Geometry: final body of the model. Coordinates: model frame, mm. Face numbers are marked on the shaded views. A direction names the side the tool comes from. Give positions to 0.01 mm unless a question says otherwise; leave off trailing zeros. Loops run counter-clockwise (first coordinate to the right, second up) from the corner with the lowest first, then second, coordinate; pieces in that order, holes last.
1. Section B-B, the plane z = 24. Output: boundary loops of the cut face in (x, y).
2. Draft query along X for the marked faces 4, 5 and 6. Return one class per face: +X half, -X half, draft (parallel to the pull), parting line (faces both ways), or undercut.
3. Section A-A, the plane y = -21. Output: boundary loops of the cut face in (x, z), then the cut area to 3 significant figures.
4. First-contact query: P1, Ø1.2, axis at x = 42.5, y = -35.5, coming from the -Z side; P2, Ø3.5, axis at x = 35, z = 34, coming from the -Y side; P3, Ø1.5, axis at x = -19.5, z = 66.5, coming from the +Y side. Flat tips, straight axial feed; report the tip coordinate or a pass-through.
5. Access query for the marked faces 1, 2 and 3. Directions: +Z, -Z, +X, -X, +Y, -Y. A direction counts if a zero-diameter tool reaches every point of the face in a straight line with its end or side. Return the directions, or none.
6. Material intervals for line 1 along Z through (x, y) = (43, -44); line 2 along Z through (x, y) = (7, -14.75); line 3 along Z through (x, y) = (40, -1.75), sorted ascending.
7. Section C-C, the plane x = -22. Output: boundary loops of the cut face in (y, z), then the cut area to 3 significant figures.
8. Section D-D, the plane z = 55. Output: boundary loops of the cut face in (x, y).
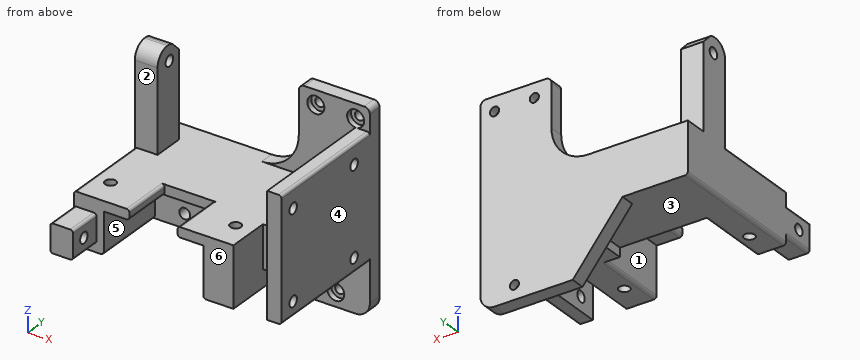
from build123d import *

# Parameters (mm, degrees)
PAD_DEPTH            = 70
SKETCH001_W          = 11.887794
SKETCH001_H          = 46.78
POCKET_DEPTH         = 70.001
POCKET001_DEPTH      = 30
SKETCH003_R          = 1.9
POCKET002_DEPTH      = 40.001
SKETCH004_W          = 17
SKETCH004_H          = 23.314381
POCKET003_DEPTH      = 40.001
SKETCH005_W          = 35
SKETCH005_H          = 57.974789
POCKET004_DEPTH      = 26
SKETCH006_W          = 45.255611
SKETCH006_H          = 30.428207
POCKET005_DEPTH      = 28
POCKET005_DEPTH_BACK = -100
SKETCH007_W          = 26.242121
SKETCH007_H          = 29.741062
POCKET006_DEPTH      = 45
SKETCH008_W          = 15.625622
SKETCH008_H          = 14.392597
SKETCH008_W_2        = 24.610352
SKETCH008_H_2        = 31.67345
POCKET007_DEPTH      = 45
SKETCH009_R          = 1.9
POCKET008_DEPTH      = 13
SKETCH010_R          = 1.6
POCKET009_DEPTH      = 5
SKETCH014_W          = 10
SKETCH014_H          = 15
PAD001_DEPTH         = 23
SKETCH015_W          = 11
SKETCH015_H          = 38.184422
SKETCH015_W_2        = 19.881198
SKETCH015_H_2        = 10
PAD002_DEPTH         = 8
SKETCH013_R          = 1.9
POCKET010_DEPTH      = 17
SKETCH011_R          = 1.9
POCKET011_DEPTH      = 15
PAD003_DEPTH         = 5
SKETCH017_R          = 3
POCKET012_DEPTH      = 2
CHAMFER_SIZE         = 4
FILLET_R             = 5
FILLET001_R          = 1
FILLET002_R          = 1
FILLET003_R          = 1
FILLET004_R          = 1
FILLET005_R          = 5
FILLET006_R          = 1
FILLET007_R          = 2
FILLET008_R          = 1
FILLET009_R          = 13
FILLET010_R          = 1
FILLET011_R          = 3


with BuildPart() as part:
    # Sketch → Pad (new body)
    with BuildSketch(Plane.XY):
        Polygon((0, 0), (45, 0), (45, -50), (-28, -50), (-28, 0), align=None)
    extrude(amount=PAD_DEPTH)

    # Sketch001 (on Face7 of Pad) → Pocket (cut, through all)
    with BuildSketch(Plane.XY.offset(70)):
        with Locations((34.056103, -28.39)):
            Rectangle(SKETCH001_W, SKETCH001_H)
    extrude(amount=-POCKET_DEPTH, mode=Mode.SUBTRACT)

    # Sketch002 (on Face5 of Pocket) → Pocket001 (cut)
    with BuildSketch(Plane.XY.offset(70)):
        Polygon((30, -5), (30, -65.096024), (-40.783405, -65.096024), (-40.783405, 12.994774), (20, 12.994774), (20, -5), align=None)
    extrude(amount=-POCKET001_DEPTH, mode=Mode.SUBTRACT)

    # Sketch003 (on Face6 of Pocket001) → Pocket002 (cut, through all)
    with BuildSketch(Plane.XY.offset(40)):
        with Locations((-22, -40)):
            Circle(SKETCH003_R)
        with Locations((22, -40)):
            Circle(SKETCH003_R)
    extrude(amount=-POCKET002_DEPTH, mode=Mode.SUBTRACT)

    # Sketch004 (on Face6 of Pocket002) → Pocket003 (cut, through all)
    with BuildSketch(Plane.XY.offset(40)):
        with Locations((0, -43.65719)):
            Rectangle(SKETCH004_W, SKETCH004_H)
    extrude(amount=-POCKET003_DEPTH, mode=Mode.SUBTRACT)

    # Sketch005 (on Face13 of Pocket003) → Pocket004 (cut)
    with BuildSketch(Plane.XZ.offset(50)):
        with Locations((0, 7.512606)):
            Rectangle(SKETCH005_W, SKETCH005_H)
    extrude(amount=-POCKET004_DEPTH, mode=Mode.SUBTRACT)

    # Sketch006 (on Face11 of Pocket004) → Pocket005 (cut, two sides)
    with BuildSketch(Plane.XZ.offset(24)) as pocket005_sk:
        with Locations((-10.127806, 6.785896)):
            Rectangle(SKETCH006_W, SKETCH006_H)
    extrude(amount=-POCKET005_DEPTH, mode=Mode.SUBTRACT)
    extrude(pocket005_sk.sketch, amount=-POCKET005_DEPTH_BACK, mode=Mode.SUBTRACT)

    # Sketch007 (on Face12 of Pocket005) → Pocket006 (cut)
    with BuildSketch(Plane.XZ.offset(50)):
        with Locations((20.733142, 3.968048)):
            Rectangle(SKETCH007_W, SKETCH007_H)
    extrude(amount=-POCKET006_DEPTH, mode=Mode.SUBTRACT)

    # Sketch008 (on Face14 of Pocket006) → Pocket007 (cut)
    with BuildSketch(Plane.XZ.offset(50)):
        with Locations((42.909006, 69.196298)):
            Rectangle(SKETCH008_W, SKETCH008_H)
        with Locations((46.359665, 3.163275)):
            Rectangle(SKETCH008_W_2, SKETCH008_H_2)
    extrude(amount=-POCKET007_DEPTH, mode=Mode.SUBTRACT)

    # Sketch009 (on Face3 of Pocket007) → Pocket008 (cut)
    with BuildSketch(Plane.YZ.offset(45)):
        with Locations((-44, 55)):
            Circle(SKETCH009_R)
        with Locations((-13, 24)):
            Circle(SKETCH009_R)
        with Locations((-13, 55)):
            Circle(SKETCH009_R)
        with Locations((-44, 24)):
            Circle(SKETCH009_R)
    extrude(amount=-POCKET008_DEPTH, mode=Mode.SUBTRACT)

    # Sketch010 (on Face1 of Pocket008) → Pocket009 (cut)
    with BuildSketch(Plane(origin=(0, 0, 0), x_dir=(-1, 0, 0), z_dir=(0, 1, 0))):
        with Locations((-33, 5)):
            Circle(SKETCH010_R)
        with Locations((-40, 65)):
            Circle(SKETCH010_R)
        with Locations((-26, 65)):
            Circle(SKETCH010_R)
    extrude(amount=-POCKET009_DEPTH, mode=Mode.SUBTRACT)

    # Sketch014 (on Face4 of Pocket009) → Pad001 (join)
    with BuildSketch(Plane.YZ.offset(45)):
        with Locations((-30, 32.5)):
            Rectangle(SKETCH014_W, SKETCH014_H)
    extrude(amount=-PAD001_DEPTH)

    # Sketch015 (on Face29 of Pad001) → Pad002 (join)
    with BuildSketch(Plane(origin=(-28, 0, 0), x_dir=(0, -1, 0), z_dir=(-1, 0, 0))):
        with Locations((13.5, 54.907789)):
            Rectangle(SKETCH015_W, SKETCH015_H)
        with Locations((52.059401, 30)):
            Rectangle(SKETCH015_W_2, SKETCH015_H_2)
    extrude(amount=-PAD002_DEPTH)

    # Sketch013 (on Face19 of Pad002) → Pocket010 (cut)
    with BuildSketch(Plane.XZ.offset(24)):
        with Locations((-7, 27)):
            Circle(SKETCH013_R)
        with Locations((7, 27)):
            Circle(SKETCH013_R)
    extrude(amount=-POCKET010_DEPTH, mode=Mode.SUBTRACT)

    # Sketch011 (on Face29 of Pad002) → Pocket011 (cut)
    with BuildSketch(Plane(origin=(-28, 0, 0), x_dir=(0, -1, 0), z_dir=(-1, 0, 0))):
        with Locations((56.5, 30)):
            Circle(SKETCH011_R)
        with Locations((13, 68.5)):
            Circle(SKETCH011_R)
    extrude(amount=-POCKET011_DEPTH, mode=Mode.SUBTRACT)

    # Sketch016 (on Face1 of Pocket011) → Pad003 (join)
    with BuildSketch(Plane(origin=(0, 0, 0), x_dir=(-1, 0, 0), z_dir=(0, 1, 0))):
        Polygon((-12.5, 0), (5, 22), (-15.71, 22), align=None)
    extrude(amount=-PAD003_DEPTH)

    # Sketch017 (on Face28 of Pad003) → Pocket012 (cut)
    with BuildSketch(Plane.XZ.offset(5)):
        with Locations((26, 65)):
            Circle(SKETCH017_R)
        with Locations((33, 5)):
            Circle(SKETCH017_R)
        with Locations((40, 65)):
            Circle(SKETCH017_R)
    extrude(amount=-POCKET012_DEPTH, mode=Mode.SUBTRACT)

    # Chamfer
    chamfer_edges = [part.edges().sort_by_distance(p)[0] for p in [
        (-24, -8, 74),
    ]]
    chamfer(chamfer_edges, length=CHAMFER_SIZE)

    # Fillet
    fillet_edges = [part.edges().sort_by_distance(p)[0] for p in [
        (-24, -19, 74),
    ]]
    fillet(fillet_edges, radius=FILLET_R)

    # Fillet001
    fillet001_edges = [part.edges().sort_by_distance(p)[0] for p in [
        (-28, -34.5, 40),
    ]]
    fillet(fillet001_edges, radius=FILLET001_R)

    # Fillet002
    fillet002_edges = [part.edges().sort_by_distance(p)[0] for p in [
        (-28, -25, 22),
    ]]
    fillet(fillet002_edges, radius=FILLET002_R)

    # Fillet003
    fillet003_edges = [part.edges().sort_by_distance(p)[0] for p in [
        (-17.5, -37, 22),
    ]]
    fillet(fillet003_edges, radius=FILLET003_R)

    # Fillet004
    fillet004_edges = [part.edges().sort_by_distance(p)[0] for p in [
        (17.5, -37, 18.838579),
    ]]
    fillet(fillet004_edges, radius=FILLET004_R)

    # Fillet005
    fillet005_edges = [part.edges().sort_by_distance(p)[0] for p in [
        (45, -2.5, 0),
    ]]
    fillet(fillet005_edges, radius=FILLET005_R)

    # Fillet006
    fillet006_edges = [part.edges().sort_by_distance(p)[0] for p in [
        (45, -27.5, 19),
        (45, -27.5, 62),
    ]]
    fillet(fillet006_edges, radius=FILLET006_R)

    # Fillet007
    fillet007_edges = [part.edges().sort_by_distance(p)[0] for p in [
        (45, -2.5, 70),
        (20, -2.5, 70),
    ]]
    fillet(fillet007_edges, radius=FILLET007_R)

    # Fillet008
    fillet008_edges = [part.edges().sort_by_distance(p)[0] for p in [
        (-8.5, -41, 36.5),
        (8.5, -41, 36.5),
        (-8.5, -41, 40),
        (8.5, -41, 40),
    ]]
    fillet(fillet008_edges, radius=FILLET008_R)

    # Fillet009
    fillet009_edges = [part.edges().sort_by_distance(p)[0] for p in [
        (20, -2.5, 40),
    ]]
    fillet(fillet009_edges, radius=FILLET009_R)

    # Fillet010
    fillet010_edges = [part.edges().sort_by_distance(p)[0] for p in [
        (-28, -56, 35),
        (-20, -56, 35),
        (-20, -56, 25),
        (-28, -56, 25),
    ]]
    fillet(fillet010_edges, radius=FILLET010_R)

    # Fillet011
    fillet011_edges = [part.edges().sort_by_distance(p)[0] for p in [
        (-24, -12, 74),
    ]]
    fillet(fillet011_edges, radius=FILLET011_R)


solid = part.part
Answers below:
1. outline: (-28, -50) - (-17.5, -50) - (-17.5, -24) - (17.5, -24) - (17.5, -50) - (28.11, -50) - (28.11, -5) - (40, -5) - (40, -11.1) - (45, -11.1) - (45, 0) - (-28, 0) - close; (40, -50) - (45, -50) - (45, -45.9) - (40, -45.9) - close; (40, -42.1) - (45, -42.1) - (45, -14.9) - (40, -14.9) - close; hole circle Ø3.8 at (-22, -40); hole circle Ø3.8 at (22, -40)
2. face 4: +X half
2. face 5: undercut
2. face 6: draft
3. outline: (-28, 23) arc R1 ccw to (-27, 22) - (12.5, 22) - (12.5, 18.84) - (28.11, 18.84) - (28.11, 40) - (-27, 40) arc R1 ccw to (-28, 39) - close; (40, 19) - (44, 19) arc R1 ccw to (45, 20) - (45, 61) arc R1 ccw to (44, 62) - (40, 62) - close; hole circle Ø3.8 at (-7, 27); hole circle Ø3.8 at (7, 27)
3. area: 1,250 mm2
4. P1: stops at z = 19
4. P2: stops at y = -35
4. P3: stops at y = -8
5. face 1: -Z, -Y
5. face 2: +Z, -X, -Y
5. face 3: -Z, -X, -Y
6. line 1: z = 19 to 22.1, 25.9 to 53.1, 56.9 to 62
6. line 2: z = 22 to 25.1, 28.9 to 40
6. line 3: z = 0 to 63.4, 66.6 to 70
7. outline: (-62, 25) - (-50, 25) - (-50, 22) - (-41.9, 22) - (-41.9, 40) - (-50, 40) - (-50, 35) - (-62, 35) - close; (-38.1, 22) - (0, 22) - (0, 40) - (-8, 40) - (-8, 70) - (-11.12, 73.12) arc R3 ccw to (-13.24, 74) - (-14, 74) arc R5 ccw to (-19, 69) - (-19, 40) - (-38.1, 40) - close; hole circle Ø3.8 at (-56.5, 30); hole circle Ø3.8 at (-13, 68.5)
7. area: 1,290 mm2
8. outline: (-28, -19) - (-20, -19) - (-20, -8) - (-28, -8) - close; (20, -5) - (40, -5) - (40, -11.1) - (45, -11.1) - (45, 0) - (20, 0) - close; (40, -50) - (45, -50) - (45, -45.9) - (40, -45.9) - close; (40, -42.1) - (45, -42.1) - (45, -14.9) - (40, -14.9) - close
